from build123d import *

# Parameters (mm, degrees)
SKETCH1_W           = 2000
SKETCH1_H           = 2000
BOSS_EXTRUDE1_DEPTH = 50
SKETCH2_R           = 6
CUT_EXTRUDE1_DEPTH  = 30
SKETCH3_W           = 2000
SKETCH3_H           = 50
CUT_EXTRUDE2_DEPTH  = 250
SKETCH4_W           = 1750
SKETCH4_H           = 50
CUT_EXTRUDE3_DEPTH  = 125
SKETCH5_W           = 1750
SKETCH5_H           = 50
CUT_EXTRUDE4_DEPTH  = 125
SKETCH6_R           = 15
SKETCH6_R_2         = 7.5
CUT_EXTRUDE5_DEPTH  = 25


with BuildPart() as part:
    # Sketch1 → Boss-Extrude1 (new body)
    with BuildSketch(Plane(origin=(0, 0, 0), x_dir=(1, 0, 0), z_dir=(0, 1, 0))):
        Rectangle(SKETCH1_W, SKETCH1_H)
    extrude(amount=-BOSS_EXTRUDE1_DEPTH)

    # Sketch2 → Cut-Extrude1 (cut)
    with BuildSketch(Plane(origin=(0, 0, 0), x_dir=(1, 0, 0), z_dir=(0, 1, 0))):
        with Locations((0, -175)):
            Circle(SKETCH2_R)
        with Locations((106, 129)):
            Circle(SKETCH2_R)
    extrude(amount=-CUT_EXTRUDE1_DEPTH, mode=Mode.SUBTRACT)

    # Sketch3 → Cut-Extrude2 (cut)
    with BuildSketch(Plane.XY.offset(1000)):
        with Locations((0, -25)):
            Rectangle(SKETCH3_W, SKETCH3_H)
    extrude(amount=-CUT_EXTRUDE2_DEPTH, mode=Mode.SUBTRACT)

    # Sketch4 → Cut-Extrude3 (cut)
    with BuildSketch(Plane.ZY.offset(1000)):
        with Locations((-125, -25)):
            Rectangle(SKETCH4_W, SKETCH4_H)
    extrude(amount=-CUT_EXTRUDE3_DEPTH, mode=Mode.SUBTRACT)

    # Sketch5 → Cut-Extrude4 (cut)
    with BuildSketch(Plane(origin=(1000, 0, 0), x_dir=(0, 0, -1), z_dir=(1, 0, 0))):
        with Locations((125, -25)):
            Rectangle(SKETCH5_W, SKETCH5_H)
    extrude(amount=-CUT_EXTRUDE4_DEPTH, mode=Mode.SUBTRACT)

    # Sketch6 → Cut-Extrude5 (cut)
    with BuildSketch(Plane(origin=(0, 0, 0), x_dir=(1, 0, 0), z_dir=(0, 1, 0))):
        with Locations((-835, -710)):
            Circle(SKETCH6_R)
        with Locations((835, 960)):
            Circle(SKETCH6_R)
        with Locations((835, -710)):
            Circle(SKETCH6_R)
        with Locations((-835, 960)):
            Circle(SKETCH6_R)
        with Locations((0, -710)):
            Circle(SKETCH6_R_2)
        with Locations((0, 960)):
            Circle(SKETCH6_R_2)
        with Locations((-835, 125)):
            Circle(SKETCH6_R_2)
        with Locations((835, 125)):
            Circle(SKETCH6_R_2)
    extrude(amount=-CUT_EXTRUDE5_DEPTH, mode=Mode.SUBTRACT)


solid = part.part
Model file for the job. Use its own axes, mm. Give positions to 0.01 mm unless a question says otherwise; leave off trailing zeros. Put each result on its own line as item: value. Start each with the question number.
(1) Drill centre lines: L1, parallel to Z at x = -835, y = -14.5; L2, parallel to Z at x = 0, y = -16; L3, parallel to X at y = -14.5, z = -960. Where is each one in solid material? Low to high. Write a range as [from, to].
(2) Pull direction X, two halves, no side cores. Call faces 1 (the face through (875, -25, -113)), 2 (the face through (-875, -25, -137)), 3 (the face through (-12, 0, -137)): released by +X, released by -X, zero draft, split by the parting line, or undercut.
(3) Pin check, flat tips, straight feed: pin 1 Ø7.5 at (x, z) = (3.5, 709.5) entering from +Y; pin 2 Ø3.5 at (x, z) = (103, -128.5) entering from +Y. Stop position of each tip, or through.
Results below:
1. L1: z = [-1000, -975], [-945, -132.5], [-117.5, 695], [725, 750]
1. L2: z = [-1000, -967.5], [-952.5, 169], [181, 702.5], [717.5, 750]
1. L3: x = [-875, -850], [-820, -7.5], [7.5, 820], [850, 875]
2. face 1: released by +X
2. face 2: released by -X
2. face 3: zero draft
3. pin 1: stops at y = -25
3. pin 2: stops at y = -30
